CAD build for the part. Positions are in the model's coordinates, mm. A direction names the side the tool comes from. Coordinates: 2 decimals unless noted, no trailing zeros. Write each loop counter-clockwise with the first axis right and the second up, starting at its lowest first coordinate (ties: lowest second). Pieces come first, ordered by that corner, then holes.
```python
from build123d import *

# Parameters (mm, degrees)
SKETCH1_W           = 63.5
SKETCH1_H           = 42.01
SKETCH1_R           = 1.27
SKETCH1_R_2         = 3.175
SKETCH1_R_3         = 7
SKETCH1_W_2         = 24.9174
SKETCH1_H_2         = 2.9972
SKETCH1_W_3         = 2.9972
SKETCH1_H_3         = 6.35
BOSS_EXTRUDE1_DEPTH = 2.9972


with BuildPart() as part:
    # Sketch1 → Boss-Extrude1 (new body)
    with BuildSketch(Plane.XY):
        Rectangle(SKETCH1_W, SKETCH1_H)
        with Locations(Location((-15.5448, -15.4678, 0), (0, 0, 180))):
            Circle(SKETCH1_R, mode=Mode.SUBTRACT)
        with Locations(Location((15.4686, -15.4678, 0), (0, 0, 180))):
            Circle(SKETCH1_R, mode=Mode.SUBTRACT)
        with Locations(Location((15.4686, 15.5186, 0), (0, 0, 180))):
            Circle(SKETCH1_R, mode=Mode.SUBTRACT)
        with Locations(Location((-15.5448, 15.5186, 0), (0, 0, 180))):
            Circle(SKETCH1_R, mode=Mode.SUBTRACT)
        with Locations(Location((25.4, 12.7, 0), (0, 0, 180))):
            Circle(SKETCH1_R_2, mode=Mode.SUBTRACT)
        with Locations(Location((0, 0, 0), (0, 0, 180))):
            Circle(SKETCH1_R_3, mode=Mode.SUBTRACT)
        with Locations(Location((-25.4, 12.7, 0), (0, 0, 180))):
            Circle(SKETCH1_R_2, mode=Mode.SUBTRACT)
        with Locations((-0.0381, -18.8714)):
            Rectangle(SKETCH1_W_2, SKETCH1_H_2, mode=Mode.SUBTRACT)
        with Locations((-25.4, -12.7)):
            Rectangle(SKETCH1_W_3, SKETCH1_H_3, mode=Mode.SUBTRACT)
        with Locations((25.4, -12.7)):
            Rectangle(SKETCH1_W_3, SKETCH1_H_3, mode=Mode.SUBTRACT)
    extrude(amount=BOSS_EXTRUDE1_DEPTH)


solid = part.part
```
Item 1: Wall check: line 1 along X through (y, z) = (-14, 0.8); line 2 along Y through (x, z) = (-15.5, 1.75) (3 decimals); line 3 along Y through (x, z) = (12, 1.7) (3 decimals). Give the ranges that are in metal, low to high.
Item 2: Saw through at D-D, the plane x = -25.4. Write the cut outline in (y, z) (3 decimals).
Item 3: Saw through at A-A, the plane y = 12.7. Write the cut outline in (x, z) (3 decimals), and give its area (3 significant figures).
Item 4: Which spindle directions (+Z, -Z, +X, -X, +Y, -Y) get a long thin tool onto all of the face, cutting with end or side? Do faces 1 (the flat face through (-26.899, -13, 1)), 2 (the flat face through (-31.75, 0, 1)). Say none if no direction does.
Item 5: Saw through at B-B, the plane x = -8.5. Write the cut outline in (y, z) (3 decimals), and give its area (3 significant figures).
Item 6: Two-plate mould, pull along Y, no slides. Class faces 3 (the flat face through (0, -20.37, 1)), 4 (the flat face through (0, -21.005, 1)), 5 (the flat face through (-8, 0, 2.997)): +Y half, -Y half, draft (parallel to the pull), parting line (faces both ways), or undercut.
Item 7: Saw through at C-C, the plane y = 0. Write the cut outline in (x, z).
Working result:
1. line 1: x = -31.75 to -26.9, -23.9 to 23.9, 26.9 to 31.75
1. line 2: y = -21.005 to -16.737, -14.199 to 14.249, 16.788 to 21.005
1. line 3: y = -21.005 to -20.37, -17.373 to 21.005
2. outline: (-21.005, 0) - (-15.875, 0) - (-15.875, 2.997) - (-21.005, 2.997) - close; (-9.525, 0) - (9.525, 0) - (9.525, 2.997) - (-9.525, 2.997) - close; (15.875, 0) - (21.005, 0) - (21.005, 2.997) - (15.875, 2.997) - close
3. outline: (-31.75, 0) - (-28.575, 0) - (-28.575, 2.997) - (-31.75, 2.997) - close; (-22.225, 0) - (22.225, 0) - (22.225, 2.997) - (-22.225, 2.997) - close; (28.575, 0) - (31.75, 0) - (31.75, 2.997) - (28.575, 2.997) - close
3. area: 152 mm2
4. face 1: +Z, -Z
4. face 2: +Z, -Z, -X, +Y, -Y
5. outline: (-21.005, 0) - (-20.37, 0) - (-20.37, 2.997) - (-21.005, 2.997) - close; (-17.373, 0) - (21.005, 0) - (21.005, 2.997) - (-17.373, 2.997) - close
5. area: 117 mm2
6. face 3: undercut
6. face 4: -Y half
6. face 5: draft
7. outline: (-31.75, 0) - (-7, 0) - (-7, 3) - (-31.75, 3) - close; (7, 0) - (31.75, 0) - (31.75, 3) - (7, 3) - close
